Could you check a few things on this drawing? It's one solid part, dimensions in mm from its lowest x, y, z. Round coordinates to 2 decimals unless told otherwise and drop trailing zeros. Order: outer loops, then holes, each group sorted by start corner. A loop starts at its lowest first (then second) coordinate and runs counter-clockwise, first axis right, second up. Notation, with made-up numbers: (85, 6) -> (139, 6) arc R13 cw to (139, 15) -> close; hole circle Ø5 at (-3, 54). An arc over 180 degrees is marked (long way). Use a Markdown table: item, result. Add a question column.
(1) I want a section at A-A, the plane x = 15. Please give me the cut outline in (y, z).
(2) I want a section at C-C, the plane z = 10. Please give me the cut outline in (x, y), then the cut area to 3 significant figures.
(3) Thinking about a two-plate mould opening in X: for the marked faces 1, 2, 3 and 4, which applies, pulls with the +X half, pulls with the -X half, needs draft (parallel to the pull), parting line crosses it, or undercut?
(4) I'm going to push flat-ended pins straight in: P1, Ø6.5, axis at x = 15, z = 10, coming from the +Y side; P2, Ø1, axis at x = 25.5, z = 10, coming from the +Y side. Where does each tip first touch, or does it pass through?
(5) If I drill on probe 1 along Z at (x, y) = (15, 26); probe 2 along Z at (x, y) = (15, 4.5); probe 3 along X at (y, z) = (28.5, 7.5), over which ranges is the centre line in solid material (lowest first)?
(6) I want a section at B-B, the plane y = 9. Please give me the cut outline in (x, z), then the cut area to 3 significant figures.
(7) I want a section at D-D, the plane z = 14.5. Please give me the cut outline in (x, y).
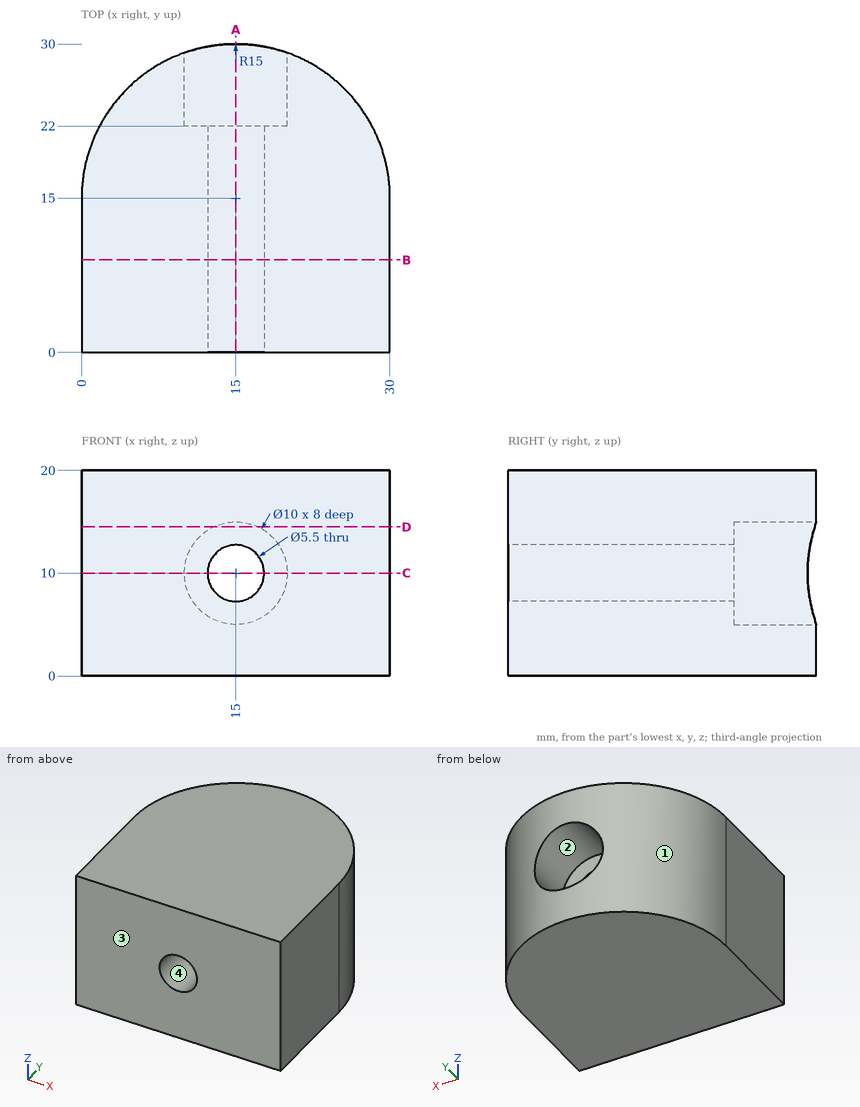
Taken from the geometry:
| question | item | result |
|---|---|---|
| 1 | outline | (0, 0) -> (30, 0) -> (30, 5) -> (22, 5) -> (22, 7.25) -> (0, 7.25) -> close; (0, 12.75) -> (22, 12.75) -> (22, 15) -> (30, 15) -> (30, 20) -> (0, 20) -> close |
| 2 | outline | (0, 0) -> (12.25, 0) -> (12.25, 22) -> (10, 22) -> (10, 29.14) arc R15 ccw to (0, 15) -> close; (17.75, 0) -> (30, 0) -> (30, 15) arc R15 ccw to (20, 29.14) -> (20, 22) -> (17.75, 22) -> close |
| 2 | area | 605 mm2 |
| 3 | face 1 | parting line crosses it |
| 3 | face 2 | undercut |
| 3 | face 3 | needs draft |
| 3 | face 4 | undercut |
| 4 | P1 | stops at y = 22 |
| 4 | P2 | stops at y = 26.18 |
| 5 | probe 1 | z = 0 to 5, 15 to 20 |
| 5 | probe 2 | z = 0 to 7.25, 12.75 to 20 |
| 5 | probe 3 | x = 8.46 to 10.67, 19.33 to 21.54 |
| 6 | outline | (0, 0) -> (30, 0) -> (30, 20) -> (0, 20) -> close; hole circle Ø5.5 at (15, 10) |
| 6 | area | 576 mm2 |
| 7 | outline | (0, 0) -> (30, 0) -> (30, 15) arc R15 ccw to (17.18, 29.84) -> (17.18, 22) -> (12.82, 22) -> (12.82, 29.84) arc R15 ccw to (0, 15) -> close |
